Check sheet for the modelled part. Datum: model origin and axes. Units: mm. A direction names the side the tool comes from. Give positions to 0.01 mm unless a question says otherwise; leave off trailing zeros. Loops run counter-clockwise (first coordinate to the right, second up) from the corner with the lowest first, then second, coordinate; pieces in that order, holes last. Notation, with made-up numbers: (10, 41.25) -> (15, 41.25) arc R12 ccw to (15, 56.25) -> close; hole circle Ø7 at (15.25, 70.5). An arc over 180 degrees is marked (long way). Answer as CSV lines item,"result". Start each with the question number.
(1) Section check A-A on z = 14. Enter the section's corners in (x, y), plus the area to 3 significant figures.
(2) Section check C-C on z = 27. Enter the section's corners in (x, y).
(3) Section check B-B on x = -3.5. Enter the section's corners in (y, z).
(4) Section check D-D on y = -16. Enter the section's corners in (x, z).
(5) Access from +Z, -Z, +X, -X, +Y, -Y to the whole of each face (thin tool, end or side, straight path). Record for faces 4 (the face through (-23.3, -11.9, 12.8)), 5 (the face through (-34, -1, 11)), 6 (the face through (14, 0, 15)).
(6) Release check for a two-part mould opening along X. For faces 1 (the face through (-12, -9.75, 53)), 2 (the face through (-15, 0, 6)), 3 (the face through (-14, 12.57, 63.27)) record: pulls with the +X half, pulls with the -X half, needs draft (parallel to the pull), parting line crosses it, or undercut.
(7) Material ranges on line 1 (Y direction, x = -24, z = 14); line 2 (Y direction, x = -20, z = 26.65); line 3 (Y direction, x = -12.5, z = 62.45), recorded low to high. Write a range as from..to.
(8) Gauge pin test, flat ends, axial feed: pin 1 Ø6.5 at (x, y) = (-32, 0) entering from +Z; pin 2 Ø1.5 at (x, z) = (-2.5, 2) entering from +Y; pin 3 Ø0.9 at (x, y) = (11.5, -11.5) entering from +Z; pin 4 Ø23.5 at (y, z) = (6, 20) entering from -X. Record the tip position at first contact, or that the pin passes through.
from build123d import *

# Parameters (mm, degrees)
SKETCH1_W                = 30
SKETCH1_H                = 30
BOSS_EXTRUDE1_DEPTH      = 65
SKETCH2_R                = 24.75
BOSS_EXTRUDE2_DEPTH      = 3
SKETCH3_R                = 23.75
CUT_EXTRUDE1_DEPTH       = 1.6
CUT_EXTRUDE4_REACH       = 74.42
SKETCH4_R                = 13.25
SKETCH5_R                = 13.75
CUT_EXTRUDE5_DEPTH       = 61
CUT_EXTRUDE9_REACH       = 82.11
CUT_EXTRUDE9_END_RADIUS  = 13.75
SKETCH8_W                = 10
SKETCH8_H                = 20
BOSS_EXTRUDE3_DEPTH      = 10
BOSS_EXTRUDE4_DEPTH      = 18.5
CUT_EXTRUDE10_REACH      = 71.346
SKETCH10_R               = 2
CUT_EXTRUDE11_REACH      = 82.11
CUT_EXTRUDE11_END_RADIUS = 13.75
CUT_EXTRUDE12_REACH      = 81.679
SKETCH13_W               = 15
SKETCH13_H               = 7
SKETCH14_W               = 11.25
SKETCH14_H               = 20
BOSS_EXTRUDE5_DEPTH      = 10
SKETCH15_W               = 21.25
SKETCH15_H               = 5
BOSS_EXTRUDE6_DEPTH      = 10
SKETCH16_W               = 10
SKETCH16_H               = 21.25
BOSS_EXTRUDE7_DEPTH      = 5
SKETCH18_R               = 2.5
CUT_EXTRUDE13_DEPTH      = 5.5
SKETCH19_R               = 1.5
CUT_EXTRUDE14_DEPTH      = 3.5
SKETCH20_R               = 1.5
CUT_EXTRUDE15_DEPTH      = 3.5


with BuildPart() as part:
    # Sketch1 → Boss-Extrude1 (new body)
    with BuildSketch(Plane.XY):
        Rectangle(SKETCH1_W, SKETCH1_H)
    extrude(amount=BOSS_EXTRUDE1_DEPTH)

    # Sketch2 → Boss-Extrude2 (add)
    with BuildSketch(Plane(origin=(0, 0, 0), x_dir=(-1, 0, 0), z_dir=(0, 0, -1))):
        Circle(SKETCH2_R)
    extrude(amount=-BOSS_EXTRUDE2_DEPTH)

    # Sketch3 → Cut-Extrude1 (cut)
    with BuildSketch(Plane(origin=(0, 0, 0), x_dir=(-1, 0, 0), z_dir=(0, 0, -1))):
        Circle(SKETCH3_R)
    extrude(amount=-CUT_EXTRUDE1_DEPTH, mode=Mode.SUBTRACT)

    # Sketch4 → Cut-Extrude4 (cut, up to next)
    with BuildSketch(Plane(origin=(0, 0, 1.6), x_dir=(-1, 0, 0), z_dir=(0, 0, -1)), mode=Mode.PRIVATE) as cut_extrude4_sk1:
        Circle(SKETCH4_R)
    cut_extrude4_tool1 = extrude(cut_extrude4_sk1.sketch, amount=-CUT_EXTRUDE4_REACH, mode=Mode.PRIVATE) & part.part
    add(cut_extrude4_tool1.solids().sort_by_distance((0, 0, 1.6))[0], mode=Mode.SUBTRACT)

    # Sketch5 → Cut-Extrude5 (cut)
    with BuildSketch(Plane.XY.offset(65)):
        Circle(SKETCH5_R)
    extrude(amount=-CUT_EXTRUDE5_DEPTH, mode=Mode.SUBTRACT)

    # Cut-Extrude9: up to this cylinder (the profile starts outside it)
    cut_extrude9_end = Plane(origin=(0, 0, 42.25), z_dir=(0, 0, 1)) * Cylinder(CUT_EXTRUDE9_END_RADIUS, 192.72, mode=Mode.PRIVATE)
    # Sketch6 → Cut-Extrude9 (cut, up to the surface)
    with BuildSketch(Plane(origin=(15, 0, 0), x_dir=(0, 0, -1), z_dir=(1, 0, 0)), mode=Mode.PRIVATE) as cut_extrude9_sk1:
        with BuildLine():
            Line((-19.5, -4.5), (-65, -4.5))
            ThreePointArc((-65, -4.5), (-69.5, 0), (-65, 4.5))
            Line((-65, 4.5), (-19.5, 4.5))
            ThreePointArc((-19.5, 4.5), (-15, 0), (-19.5, -4.5))
        make_face()
    cut_extrude9_tool1 = extrude(cut_extrude9_sk1.sketch, amount=-CUT_EXTRUDE9_REACH, mode=Mode.PRIVATE) - cut_extrude9_end
    add(cut_extrude9_tool1.solids().sort_by_distance((15, 0, 42.25))[0], mode=Mode.SUBTRACT)

    # Sketch8 → Boss-Extrude3 (add)
    with BuildSketch(Plane.ZY.offset(15)):
        with Locations((14, 0)):
            Rectangle(SKETCH8_W, SKETCH8_H)
    extrude(amount=BOSS_EXTRUDE3_DEPTH)

    # Sketch9 → Boss-Extrude4 (add)
    with BuildSketch(Plane.ZY.offset(25)):
        with BuildLine():
            Line((17, 3), (17, -3))
            ThreePointArc((17, -3), (14, -6), (11, -3))
            Line((11, -3), (11, 3))
            ThreePointArc((11, 3), (14, 6), (17, 3))
        make_face()
    extrude(amount=BOSS_EXTRUDE4_DEPTH)

    # Sketch10 → Cut-Extrude10 (cut, up to next)
    with BuildSketch(Plane.XY.offset(17), mode=Mode.PRIVATE) as cut_extrude10_sk1:
        with Locations((-40.5, 0)):
            Circle(SKETCH10_R)
    cut_extrude10_tool1 = extrude(cut_extrude10_sk1.sketch, amount=-CUT_EXTRUDE10_REACH, mode=Mode.PRIVATE) & part.part
    # Sketch10 → Cut-Extrude10 (cut, up to next)
    with BuildSketch(Plane.XY.offset(17), mode=Mode.PRIVATE) as cut_extrude10_sk2:
        with Locations((-32, 0)):
            Circle(SKETCH10_R)
    cut_extrude10_tool2 = extrude(cut_extrude10_sk2.sketch, amount=-CUT_EXTRUDE10_REACH, mode=Mode.PRIVATE) & part.part
    add(cut_extrude10_tool1.solids().sort_by_distance((-40.5, 0, 17))[0], mode=Mode.SUBTRACT)
    add(cut_extrude10_tool2.solids().sort_by_distance((-32, 0, 17))[0], mode=Mode.SUBTRACT)

    # Cut-Extrude11: up to this cylinder (the profile starts outside it)
    cut_extrude11_end = Plane(origin=(0, 0, 52.5), z_dir=(0, 0, 1)) * Cylinder(CUT_EXTRUDE11_END_RADIUS, 192.72, mode=Mode.PRIVATE)
    # Sketch11 → Cut-Extrude11 (cut, up to the surface)
    with BuildSketch(Plane.ZY.offset(15), mode=Mode.PRIVATE) as cut_extrude11_sk1:
        with BuildLine():
            Line((40, 9.75), (65, 9.75))
            ThreePointArc((65, 9.75), (74.75, 0), (65, -9.75))
            Line((65, -9.75), (40, -9.75))
            ThreePointArc((40, -9.75), (30.25, 0), (40, 9.75))
        make_face()
    cut_extrude11_tool1 = extrude(cut_extrude11_sk1.sketch, amount=-CUT_EXTRUDE11_REACH, mode=Mode.PRIVATE) - cut_extrude11_end
    add(cut_extrude11_tool1.solids().sort_by_distance((-15, 0, 52.5))[0], mode=Mode.SUBTRACT)

    # Sketch13 → Cut-Extrude12 (cut, up to next)
    with BuildSketch(Plane.XY.offset(3), mode=Mode.PRIVATE) as cut_extrude12_sk1:
        with Locations((0, -18.5)):
            Rectangle(SKETCH13_W, SKETCH13_H)
    cut_extrude12_tool1 = extrude(cut_extrude12_sk1.sketch, amount=-CUT_EXTRUDE12_REACH, mode=Mode.PRIVATE) & part.part
    add(cut_extrude12_tool1.solids().sort_by_distance((0, -18.5, 3))[0], mode=Mode.SUBTRACT)

    # Sketch14 → Boss-Extrude5 (add)
    with BuildSketch(Plane.ZY.offset(15)):
        with Locations((24.625, 0)):
            Rectangle(SKETCH14_W, SKETCH14_H)
    extrude(amount=BOSS_EXTRUDE5_DEPTH)

    # Sketch15 → Boss-Extrude6 (add)
    with BuildSketch(Plane.ZY.offset(15)):
        with Locations((19.625, 12.5)):
            Rectangle(SKETCH15_W, SKETCH15_H)
    extrude(amount=BOSS_EXTRUDE6_DEPTH)

    # Sketch16 → Boss-Extrude7 (add)
    with BuildSketch(Plane(origin=(0, -10, 0), x_dir=(-1, 0, 0), z_dir=(0, -1, 0))):
        with Locations((20, -19.625)):
            Rectangle(SKETCH16_W, SKETCH16_H)
    extrude(amount=BOSS_EXTRUDE7_DEPTH)

    # Sketch18 → Cut-Extrude13 (cut)
    with BuildSketch(Plane.XY.offset(30.25)):
        with Locations((-20, -11)):
            Circle(SKETCH18_R)
        with Locations((-20, 11)):
            Circle(SKETCH18_R)
    extrude(amount=-CUT_EXTRUDE13_DEPTH, mode=Mode.SUBTRACT)

    # Sketch19 → Cut-Extrude14 (cut)
    with BuildSketch(Plane.XY.offset(65)):
        with Locations((12, -12)):
            Circle(SKETCH19_R)
        with Locations((12, 12)):
            Circle(SKETCH19_R)
        with Locations((-12.5, -12.5)):
            Circle(SKETCH19_R)
        with Locations((-12.5, 12.5)):
            Circle(SKETCH19_R)
    extrude(amount=-CUT_EXTRUDE14_DEPTH, mode=Mode.SUBTRACT)

    # Sketch20 → Cut-Extrude15 (cut)
    with BuildSketch(Plane.ZY.offset(25)):
        with Locations((14, 11)):
            Circle(SKETCH20_R)
        with Locations((14, -11)):
            Circle(SKETCH20_R)
    extrude(amount=-CUT_EXTRUDE15_DEPTH, mode=Mode.SUBTRACT)


solid = part.part
Working result:
1,outline,"(-43.5, -6) -> (-25, -6) -> (-25, -9.5) -> (-21.5, -9.5) -> (-21.5, -12.5) -> (-25, -12.5) -> (-25, -15) -> (15, -15) -> (15, 15) -> (-25, 15) -> (-25, 12.5) -> (-21.5, 12.5) -> (-21.5, 9.5) -> (-25, 9.5) -> (-25, 6) -> (-43.5, 6) -> close; hole circle Ø4 at (-40.5, 0); hole circle Ø4 at (-32, 0); hole circle Ø27.5 at (0, 0)"
1,area,"782 mm^2"
2,outline,"(-25, -15) -> (15, -15) -> (15, -4.5) -> (12.99, -4.5) arc R13.75 cw (long way) to (12.99, 4.5) -> (15, 4.5) -> (15, 15) -> (-25, 15) -> close; hole circle Ø5 at (-20, -11); hole circle Ø5 at (-20, 11)"
3,outline,"(-24.5, 0) -> (-23.49, 0) -> (-23.49, 1.6) -> (-22, 1.6) -> (-22, 3) -> (-24.5, 3) -> close; (-15, 1.6) -> (-12.78, 1.6) -> (-12.78, 4) -> (-13.3, 4) -> (-13.3, 65) -> (-15, 65) -> close; (12.78, 1.6) -> (23.49, 1.6) -> (23.49, 0) -> (24.5, 0) -> (24.5, 3) -> (15, 3) -> (15, 65) -> (13.3, 65) -> (13.3, 4) -> (12.78, 4) -> close"
4,outline,"(-18.88, 0) -> (-17.55, 0) -> (-17.55, 1.6) -> (-7.5, 1.6) -> (-7.5, 3) -> (-18.88, 3) -> close; (7.5, 1.6) -> (17.55, 1.6) -> (17.55, 0) -> (18.88, 0) -> (18.88, 3) -> (7.5, 3) -> close"
5,face 4,"-X"
5,face 5,"-Z, -X, +Y, -Y"
5,face 6,"+Z, +X"
6,face 1,"needs draft"
6,face 2,"pulls with the -X half"
6,face 3,"undercut"
7,line 1,"y = -15..-12.5, -9.5..9.5, 12.5..15"
7,line 2,"y = -15..-13.5, -8.5..8.5, 13.5..15"
7,line 3,"y = -15..-14, -11..-9.75, 9.75..11, 14..15"
8,pin 1,"stops at z = 17"
8,pin 2,"stops at y = 24.69"
8,pin 3,"stops at z = 61.5"
8,pin 4,"stops at x = -43.5"
